Design review of the part shown in the three views and the two pictorial views. Dimensions are in mm from the part's minimum x, y and z. A direction names the side the tool comes from. Coordinates: 2 decimals unless noted, no trailing zeros. Order: outer loops, then holes, each group sorted by start corner. A loop starts at its lowest first (then second) coordinate and runs counter-clockwise, first axis right, second up. Notation, with made-up numbers: (27, 5) -> (73, 5) arc R19 ccw to (73, 31) -> close; hole circle Ø11 at (-26.75, -10). An arc over 180 degrees is marked (long way). Answer as a JSON object with one key per item and string values. Group by question number.
1) Add section A-A, the plane z = 1. Write out the cut boundary in (x, y).
2) Wall thickness on L1, parallel to X at y = 23.75, z = 5.5; L2, parallel to Y at x = 7.25, z = 2: over which ranges is each line inside the solid? List them lowest first.
3) Machinability: for the marked faces 1, 2, 3, 4 and 5, which of the approach directions +Z, -Z, +X, -X, +Y, -Y give a long, thin tool a straight path to every point of the face, cutting with its end or side? Answer none if there is none.
4) Add section B-B, the plane y = 13.5. Write out the cut boundary in (x, z).
5) For pin 1 (3 mm diameter, centred on y = 23.5, z = 6.5, fed in from -X); pin 2 (2.5 mm diameter, centred on y = 12.5, z = 1.5, fed in from +X); pin 3 (1.8 mm diameter, centred on y = 17.5, z = 7, fed in from +X), all flat-tipped, find the tip position at first contact; note any pin that passes through.
6) Add section D-D, the plane z = 7.25. Write out the cut boundary in (x, y).
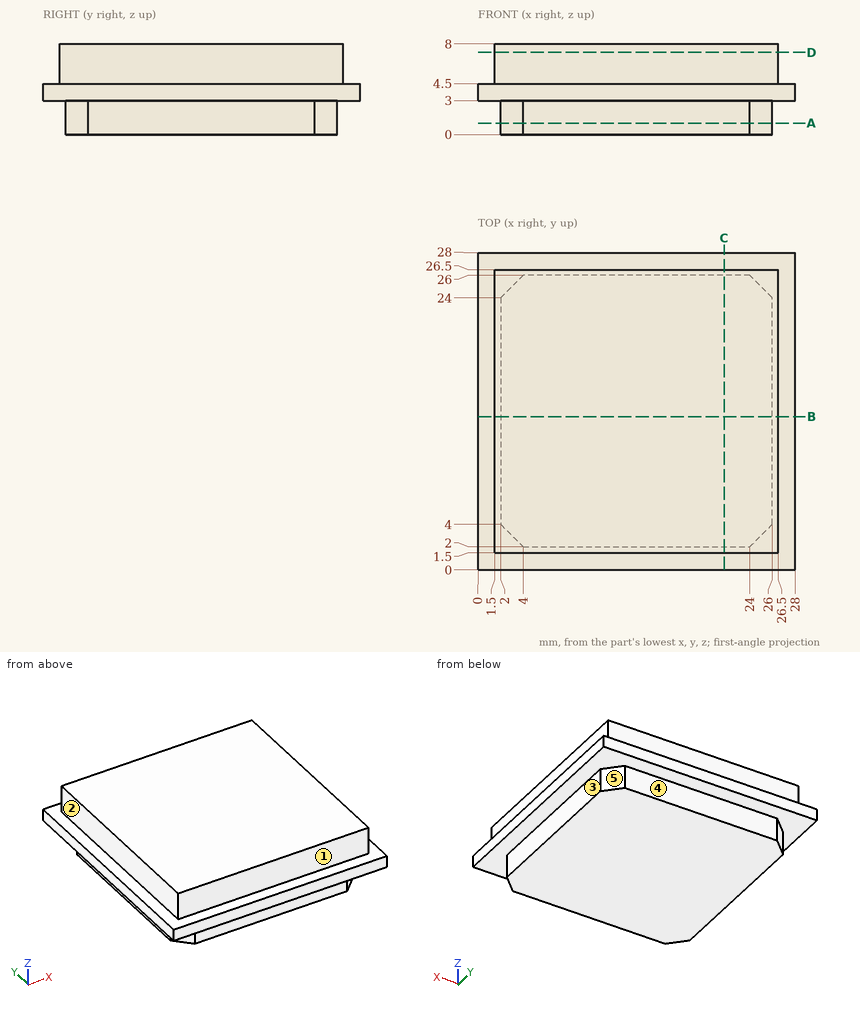
Output values:
{
 "1": {"outline": "(2, 4) -> (4, 2) -> (24, 2) -> (26, 4) -> (26, 24) -> (24, 26) -> (4, 26) -> (2, 24) -> close"},
 "2": {"L1": "x = 1.5 to 26.5", "L2": "y = 2 to 26"},
 "3": {"face 1": "+Z, +X, -X, -Y", "face 2": "+Z, -X, +Y, -Y", "face 3": "-Z, +X, +Y, -Y", "face 4": "-Z, +X, -X, +Y", "face 5": "-Z, +X, +Y"},
 "4": {"outline": "(0, 3) -> (2, 3) -> (2, 0) -> (26, 0) -> (26, 3) -> (28, 3) -> (28, 4.5) -> (26.5, 4.5) -> (26.5, 8) -> (1.5, 8) -> (1.5, 4.5) -> (0, 4.5) -> close"},
 "5": {"pin 1": "stops at x = 1.5", "pin 2": "stops at x = 26", "pin 3": "stops at x = 26.5"},
 "6": {"outline": "(1.5, 1.5) -> (26.5, 1.5) -> (26.5, 26.5) -> (1.5, 26.5) -> close"}
}
